from build123d import *

# Parameters (mm, degrees)
F0_W     = 150
F0_H     = 160
F1_DEPTH = 10
F2_W     = 150
F2_H     = 160
F2_W_2   = 140
F2_H_2   = 150
F3_DEPTH = 30
F4_W     = 140
F4_H     = 150
F4_W_2   = 40.476516
F4_H_2   = 6
F4_H_3   = 5
F4_H_4   = 15
F4_H_5   = 11
F4_H_6   = 12
F4_H_7   = 7
F5_DEPTH = 10


with BuildPart() as f1:
    # F0 (on Top) → F1 (new body)
    with BuildSketch(Plane.XY):
        Rectangle(F0_W, F0_H)
    extrude(amount=F1_DEPTH)

    # F2 (on face) → F3 (join)
    with BuildSketch(Plane.XY.offset(10)):
        Rectangle(F2_W, F2_H)
        Rectangle(F2_W_2, F2_H_2, mode=Mode.SUBTRACT)
    extrude(amount=F3_DEPTH)

    # F4 (on face) → F5 (join)
    with BuildSketch(Plane.XY.offset(10)):
        Rectangle(F4_W, F4_H)
        with Locations((44.761742, -67)):
            Rectangle(F4_W_2, F4_H_2, mode=Mode.SUBTRACT)
        with Locations((44.761742, -58.5)):
            Rectangle(F4_W_2, F4_H_3, mode=Mode.SUBTRACT)
        with Locations((44.761742, -47)):
            Rectangle(F4_W_2, F4_H_2, mode=Mode.SUBTRACT)
        with Locations((44.761742, -32)):
            Rectangle(F4_W_2, F4_H_2, mode=Mode.SUBTRACT)
        with Locations((44.761742, -22.5)):
            Rectangle(F4_W_2, F4_H_3, mode=Mode.SUBTRACT)
        with Locations((44.761742, -12)):
            Rectangle(F4_W_2, F4_H_2, mode=Mode.SUBTRACT)
        with Locations((44.761742, -2)):
            Rectangle(F4_W_2, F4_H_2, mode=Mode.SUBTRACT)
        with Locations((44.761742, 8)):
            Rectangle(F4_W_2, F4_H_2, mode=Mode.SUBTRACT)
        with Locations((44.761742, 22.5)):
            Rectangle(F4_W_2, F4_H_4, mode=Mode.SUBTRACT)
        with Locations((44.761742, 40.5)):
            Rectangle(F4_W_2, F4_H_5, mode=Mode.SUBTRACT)
        with Locations((44.761742, 56)):
            Rectangle(F4_W_2, F4_H_6, mode=Mode.SUBTRACT)
        with Locations((44.761742, 68.5)):
            Rectangle(F4_W_2, F4_H_7, mode=Mode.SUBTRACT)
    extrude(amount=F5_DEPTH)


solid = f1.part
The listing builds one solid part. Answer for the finished solid, in the listing's coordinates (mm). Coordinates: 2 decimals unless noted, no trailing zeros. Write each loop counter-clockwise with the first axis right and the second up, starting at its lowest first coordinate (ties: lowest second). Pieces come first, ordered by that corner, then holes. Notation, with made-up numbers: M -1,24.25 L 7,24.25 A23 ccw 7,53.25 Z; hole C 71.5,-16.75 d4. An arc over 180 degrees is marked long. Use one line per item in the form item = value.
Item 1: Find section C-C, the plane x = -58. Give the vertices of the cut face in (y, z), plus the area to 3 significant figures.
Model answer:
outline = M -80,0 L 80,0 L 80,40 L 75,40 L 75,20 L -75,20 L -75,40 L -80,40 Z
area = 3,400 mm2
Item 2: Find section B-B, the plane y = 56. Give the vertices of the cut face in (x, z).
Model answer:
outline = M -75,0 L 75,0 L 75,40 L 70,40 L 70,20 L 65,20 L 65,10 L 24.52,10 L 24.52,20 L -70,20 L -70,40 L -75,40 Z
Item 3: Given P1, Ø1.8, axis at x = 52, y = 7.5, coming from the +Z side, flat-ended and moving along its own axis, determine where the tip first touches the part or whether it passes through.
Model answer:
P1 = 10
Item 4: The mould has two halves that part along X. Classify faces 1 (the face through (-1, -80, 20)), 2 (the face through (44, -35, 15)), 3 (the face through (-75, -1, 20)): released by +X, released by -X, zero draft, split by the parting line, or undercut.
Model answer:
face_1 = zero draft
face_2 = undercut
face_3 = released by -X
Item 5: Find the intervals of material crossed by probe 1 along X at (y, z) = (35.5, 32.5); probe 2 along Y at (x, z) = (14, 38); probe 3 along X at (y, z) = (58, 12.5), in increasing order.
Model answer:
probe_1 = -75 to -70, 70 to 75
probe_2 = -80 to -75, 75 to 80
probe_3 = -75 to 24.52, 65 to 75
Item 6: Find section D-D, the plane z = 14.5. Give the number of separate pieces and of enclosed holes in the cut face, plus the area to 3 significant figures.
Model answer:
separate_pieces = 1
enclosed_holes = 12
area = 20,300 mm2
Item 7: Find section A-A, the plane z = 23.5. Give the vertices of the cut face in (x, y), plus the area to 3 significant figures.
Model answer:
outline = M -75,-80 L 75,-80 L 75,80 L -75,80 Z; hole M -70,-75 L 70,-75 L 70,75 L -70,75 Z
area = 3,000 mm2
